from build123d import *

# Parameters (mm, degrees)
BOSS_EXTRUDE1_DEPTH = 20
SKETCH2_R           = 1.75
SKETCH2_R_2         = 4.5
CUT_EXTRUDE1_DEPTH  = 3.9
SKETCH3_R           = 0.75
BOSS_EXTRUDE2_DEPTH = 1.5
FILLET1_R           = 2
CUT_EXTRUDE2_DEPTH  = 1


with BuildPart() as part:
    # Sketch1 → Boss-Extrude1 (new body)
    with BuildSketch(Plane.XY):
        Polygon((0, 0), (0, -44), (2, -44), (2, -28), (2.9, -28), (2.9, -16), (2, -16), (2, 0), align=None)
    extrude(amount=BOSS_EXTRUDE1_DEPTH)

    # Sketch2 → Cut-Extrude1 (cut, through all)
    with BuildSketch(Plane.ZY):
        with Locations((10, -7)):
            Circle(SKETCH2_R)
        with Locations((10, -37)):
            Circle(SKETCH2_R)
        with Locations((10, -22)):
            Circle(SKETCH2_R_2)
    extrude(amount=-CUT_EXTRUDE1_DEPTH, mode=Mode.SUBTRACT)

    # Sketch3 → Boss-Extrude2 (add)
    with BuildSketch(Plane(origin=(2.9, 0, 0), x_dir=(0, 0, -1), z_dir=(1, 0, 0))):
        with Locations((-17.5, -25.5)):
            Circle(SKETCH3_R)
        with Locations((-2.5, -18.5)):
            Circle(SKETCH3_R)
    extrude(amount=BOSS_EXTRUDE2_DEPTH)

    # Fillet1
    fillet1_edges = [part.edges().sort_by_distance(p)[0] for p in [
        (1, -44, 20),
        (1, 0, 0),
        (1, 0, 20),
        (1, -44, 0),
    ]]
    fillet(fillet1_edges, radius=FILLET1_R)

    # Sketch4 → Cut-Extrude2 (cut)
    with BuildSketch(Plane.ZY):
        Polygon((11.876388375, -10.25), (13.75277675, -7), (11.876388375, -3.75), (8.123611625, -3.75), (6.24722325, -7), (8.123611625, -10.25), align=None)
        Polygon((11.876388375, -40.25), (13.75277675, -37), (11.876388375, -33.75), (8.123611625, -33.75), (6.24722325, -37), (8.123611625, -40.25), align=None)
    extrude(amount=-CUT_EXTRUDE2_DEPTH, mode=Mode.SUBTRACT)


solid = part.part
CAD build for the part. Positions are in the model's coordinates, mm. A direction names the side the tool comes from. Give positions to 0.01 mm unless a question says otherwise; leave off trailing zeros. Order: outer loops, then holes, each group sorted by start corner. A loop starts at its lowest first (then second) coordinate and runs counter-clockwise, first axis right, second up. Notation, with made-up numbers: (-18.5, 87.5) - (0.5, 87.5) arc R30 ccw to (0.5, 123.5) - close; hole circle Ø11 at (55.5, -33.5). An arc over 180 degrees is marked (long way). Answer in a Markdown table with one row per item.
1. Flat gauge pins, fed straight in: pin 1 (0.7 mm diameter, centred on x = 2.5, z = 13.5, fed in from -Y); pin 2 (5 mm diameter, centred on y = -37.5, z = 11, fed in from -X); pin 3 (4 mm diameter, centred on y = -23, z = 5.5, fed in from +X); pin 4 (3 mm diameter, centred on y = -7, z = 10, fed in from +X). Where does each tip first touch, or does it go through?
Data:
| item | result |
|---|---|
| pin 1 | stops at y = -28 |
| pin 2 | stops at x = 0 |
| pin 3 | stops at x = 2.9 |
| pin 4 | passes through |
2. Saw through at D-D, the plane z = 16. Give the cut face in (x, y), plus the area to 3 significant figures.
Data:
| item | result |
|---|---|
| outline | (0, -44) - (2, -44) - (2, -28) - (2.9, -28) - (2.9, -16) - (2, -16) - (2, 0) - (0, 0) - close |
| area | 98.8 mm² |
3. Saw through at A-A, the plane y = -22. Give the cut face in (x, z).
Data:
| item | result |
|---|---|
| outline | (0, 0) - (2.9, 0) - (2.9, 5.5) - (0, 5.5) - close; (0, 14.5) - (2.9, 14.5) - (2.9, 20) - (0, 20) - close |
4. Pull direction Z, two halves, no side cores. Call faces 1 (the flat face through (0, -22, 5)), 2 (the cylindrical face through (1.01, -43.4, 19.43)), 3 (the flat face through (0.5, -33.75, 10)), 4 (the flat face through (0.49, -5.35, 7.2)): pulls with the +Z half, pulls with the -Z half, needs draft (parallel to the pull), parting line crosses it, or undercut.
Data:
| item | result |
|---|---|
| face 1 | needs draft |
| face 2 | pulls with the +Z half |
| face 3 | undercut |
| face 4 | undercut |
5. Saw through at C-C, the plane x = 3.85. Give the cut face in (y, z), plus the area to 3 significant figures.
Data:
| item | result |
|---|---|
| outline | circle Ø1.5 at (-25.5, 17.5); circle Ø1.5 at (-18.5, 2.5) |
| area | 3.53 mm² |
6. Tool access for faces 5 (the flat face through (0.5, -10.25, 10)), 6 (the flat face through (2.5, -16, 9.9)), 7 (the flat face through (4.4, -18.5, 2.5)): list every direction of +Z, -Z, +X, -X, +Y, -Y with a clear straight run to the whole face (end or side of a thin tool).
Data:
| item | result |
|---|---|
| face 5 | -X |
| face 6 | +Z, -Z, +X, +Y |
| face 7 | +Z, -Z, +X, +Y, -Y |
7. Probe probe 1 along Y at (x, z) = (0.85, 10); probe 2 along Y at (x, z) = (1.25, 10); probe 3 along X at (y, z) = (-33.5, 16). List the from-to ranges inside material, lowest first. Write a range as [from, to].
Data:
| item | result |
|---|---|
| probe 1 | y = [-44, -40.25], [-33.75, -26.5], [-17.5, -10.25], [-3.75, 0] |
| probe 2 | y = [-44, -38.75], [-35.25, -26.5], [-17.5, -8.75], [-5.25, 0] |
| probe 3 | x = [0, 2] |
8. Saw through at B-B, the plane z = 10.5. Give the cut face in (x, y).
Data:
| item | result |
|---|---|
| outline | (0, -44) - (2, -44) - (2, -38.68) - (1, -38.68) - (1, -40.25) - (0, -40.25) - close; (0, -33.75) - (1, -33.75) - (1, -35.32) - (2, -35.32) - (2, -28) - (2.9, -28) - (2.9, -26.47) - (0, -26.47) - close; (0, -17.53) - (2.9, -17.53) - (2.9, -16) - (2, -16) - (2, -8.68) - (1, -8.68) - (1, -10.25) - (0, -10.25) - close; (0, -3.75) - (1, -3.75) - (1, -5.32) - (2, -5.32) - (2, 0) - (0, 0) - close |
